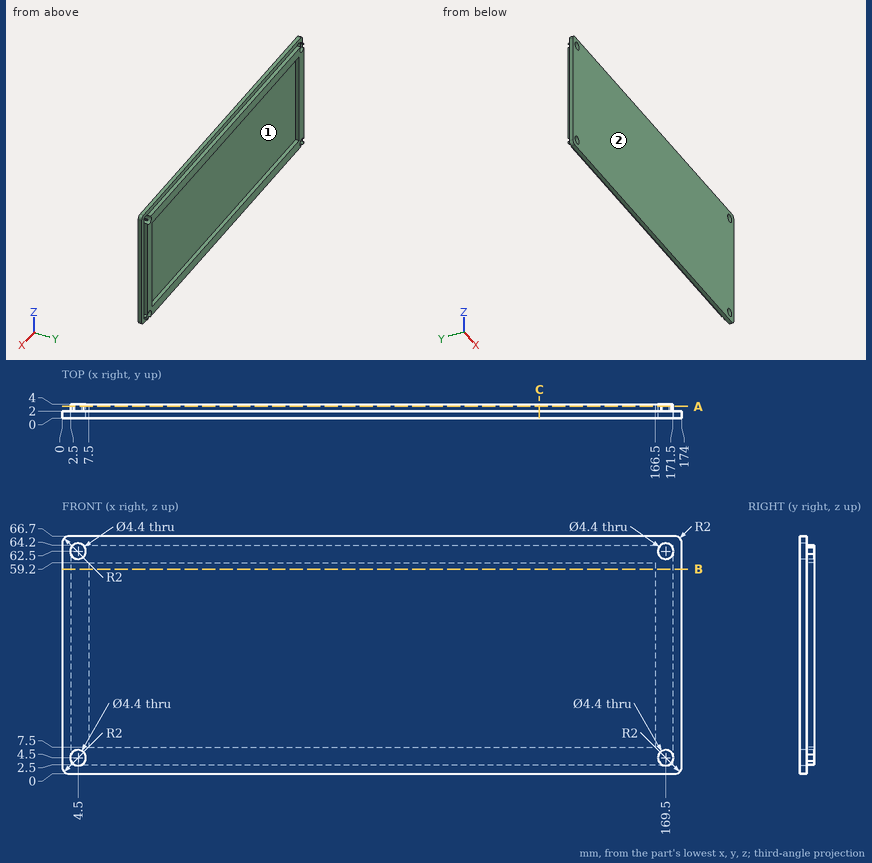
Print and shaded views of the part. All mm, measured from the part's lowest x, y and z. Round coordinates to 2 decimals unless told otherwise and drop trailing zeros. Write each loop counter-clockwise with the first axis right and the second up, starting at its lowest first coordinate (ties: lowest second). Pieces come first, ordered by that corner, then holes. Notation, with made-up numbers: (43.25, 58.25) - (67.25, 58.25) arc R9 ccw to (67.25, 70.25) - close; hole circle Ø6 at (79, 5.25). An arc over 180 degrees is marked (long way). One line per question, with ' | ' between items.
1. Band-saw the part on B-B, the plane z = 57.5. Write the cut outline in (x, y), and give its area (3 significant figures).
Results are:
outline: (0, 0) - (174, 0) - (174, 2) - (171.5, 2) - (171.5, 4) - (166.5, 4) - (166.5, 2) - (7.5, 2) - (7.5, 4) - (2.5, 4) - (2.5, 2) - (0, 2) - close | area: 368 mm^2
2. Band-saw the part on C-C, the plane x = 134. Write the cut outline in (y, z).
Results are:
outline: (0, 0) - (2, 0) - (2, 2.5) - (4, 2.5) - (4, 7.5) - (2, 7.5) - (2, 59.2) - (4, 59.2) - (4, 64.2) - (2, 64.2) - (2, 66.7) - (0, 66.7) - close
3. Mould opens along Z. For the marked faces 1 and 2 say: released by +Z, released by -Z, zero draft, split by the parting line, or undercut.
Results are:
face 1: undercut | face 2: zero draft
4. Drill centre lines: line 1 along Z through (x, y) = (169.5, 1.1); line 2 along Z through (x, y) = (63, 3.75); line 3 along X through (y, z) = (2.55, 35). Where is each one in solid material? Low to high. Write a range as from..to.
Results are:
line 1: 0..2.3, 6.7..60.3, 64.7..66.7 | line 2: 2.5..7.5, 59.2..64.2 | line 3: 2.5..7.5, 166.5..171.5
5. Drop flat-ended pins along their axis: pin 1 Ø12 at (x, z) = (37, 42) entering from +Y; pin 2 Ø0.6 at (y, z) = (3.5, 64) entering from +X; pin 3 Ø0.5 at (x, y) = (3, 3) entering from -Z. Give the stop position or say it passes through.
Results are:
pin 1: y = 2 | pin 2: x = 171.5 | pin 3: z = 2.5
6. Band-saw the part on A-A, the plane y = 3.3. Write the cut outline in (x, z), and give its area (3 significant figures).
Results are:
outline: (2.5, 2.5) - (3.58, 2.5) arc R2.2 cw to (2.5, 3.58) - close; (2.5, 5.42) arc R2.2 cw (long way) to (5.42, 2.5) - (168.58, 2.5) arc R2.2 cw (long way) to (171.5, 5.42) - (171.5, 61.58) arc R2.2 cw (long way) to (168.1, 64.2) - (5.9, 64.2) arc R2.2 cw (long way) to (2.5, 61.58) - close; (2.5, 63.42) arc R2.2 cw to (3.1, 64.2) - (2.5, 64.2) - close; (170.42, 2.5) - (171.5, 2.5) - (171.5, 3.58) arc R2.2 cw to start; (170.9, 64.2) arc R2.2 cw to (171.5, 63.42) - (171.5, 64.2) - close; hole (7.5, 7.5) - (166.5, 7.5) - (166.5, 59.2) - (7.5, 59.2) - close | area: 2,150 mm^2
